Part model, mm, in its own coordinate system. A direction names the side the tool comes from. Coordinates: 2 decimals unless noted, no trailing zeros. Loops run counter-clockwise (first coordinate to the right, second up) from the corner with the lowest first, then second, coordinate; pieces in that order, holes last. Notation, with made-up numbers: M 66.5,10.5 L 113.5,10.5 A27 ccw 113.5,27.5 Z; hole C 26.25,69.5 d2. An arc over 180 degrees is marked long. Use a Markdown table: item, result. Add a question column.
1) Pull direction Y, two halves, no side cores. Call faces 1 (the flat face through (10, 4.758, 2)), 2 (the cylindrical face through (1.6, -28.8, 2)), 3 (the flat face through (3.167, -27.731, 2.366)): released by +Y, released by -Y, zero draft, split by the parting line, or undercut.
2) Band-saw the part on D-D (x = 9.5). List the corners of the cut face in (y, z), plus the area to 3 significant figures.
3) Pin check, flat tips, straight feed: pin 1 Ø10 at (x, y) = (16, -21.5) entering from +Z; pin 2 Ø2.5 at (y, z) = (-14.5, 2) entering from +X; pin 3 Ø2.5 at (y, z) = (-15, 3.5) entering from -X; pin 4 Ø4 at (x, y) = (1.5, 1) entering from -Z. Stop position of each tip, or through.
4) Band-saw the part on A-A (x = 0). List the corners of the cut face in (y, z).
5) Band-saw the part on B-B (z = 3.1). List the corners of the cut face in (x, y).
6) Tool access for faces 4 (the flat face through (0.754, -18, 2)), 5 (the flat face through (7.88, -15, 2)), 6 (the flat face through (2.554, -27, 2)), 7 (the flat face through (7.15, -11.65, 2.37)): list every direction of +Z, -Z, +X, -X, +Y, -Y with a clear straight run to the whole face (end or side of a thin tool).
7) Wall check: probe 1 along Y at (x, z) = (14.25, 2.75); probe 2 along X at (y, z) = (-17, 4.2); probe 3 along Y at (x, z) = (1.75, 0.9). Give the ranges that are in metal, low to high. Write a range as from..to.
8) Band-saw the part on C-C (y = -16). List the corners of the cut face in (x, z).
from build123d import *

# Parameters (mm, degrees)
SKETCH_1_R          = 5
SKETCH_1_R_2        = 2.5
EXTRUDE_1_DEPTH     = 4.8
SKETCH_3_R          = 1.825
CUT_EXTRUDE_1_DEPTH = 1.8
CUT_EXTRUDE_2_REACH = 36.158
SKETCH_4_R          = 0.1


with BuildPart() as part:
    # 스케치1 → 보스-돌출1 (new body)
    # profile 1 of 2: a face of its own
    with BuildSketch(Plane.XY):
        with BuildLine():
            ThreePointArc((5, 0), (0, -5), (-5, 0))
            Line((-5, 0), (-5, -2.326474397))
            Line((-5, -2.326474397), (0.754164722, -7.377840375))
            Line((0.754164722, -7.377840375), (0.754164722, -29.519890116))
            Line((0.754164722, -29.519890116), (2.889052882, -29.519890116))
            Line((2.889052882, -29.519890116), (3.452626944, -25.890848407))
            Line((3.452626944, -25.890848407), (7.880357437, -17.740939791))
            Line((7.880357437, -17.740939791), (7.880357437, -12.211059606))
            Line((7.880357437, -12.211059606), (6.40208237, -11.079255258))
            Line((6.40208237, -11.079255258), (6.40208237, -3.237610212))
            ThreePointArc((6.40208237, -3.237610212), (6.694975589, -2.530503431), (7.40208237, -2.237610212))
            Line((7.40208237, -2.237610212), (18.063612226, -2.237610212))
            Line((18.063612226, -2.237610212), (19.056002599, 4.757997197))
            Line((19.056002599, 4.757997197), (1.536705134, 4.757997197))
            ThreePointArc((1.536705134, 4.757997197), (4.04249463, 2.942488261), (5, 0))
        make_face()
    # profile 2 of 2: a face of its own
    with BuildSketch(Plane.XY):
        Circle(SKETCH_1_R)
        Circle(SKETCH_1_R_2, mode=Mode.SUBTRACT)
    extrude(amount=EXTRUDE_1_DEPTH)

    # 스케치3 → 컷-돌출1 (cut)
    with BuildSketch(Plane.ZY.offset(-0.754164722)):
        with Locations((2.4, -27.019890116)):
            Circle(SKETCH_3_R)
    extrude(amount=-CUT_EXTRUDE_1_DEPTH, mode=Mode.SUBTRACT)

    # 컷-돌출2: up to this plane
    cut_extrude_2_end = Plane(origin=(7.297372122, -1.133249487, 4.8), z_dir=(-0.9881554576984991, 0.15345615471746255, 0))
    # 스케치4 → 컷-돌출2 (cut, up to the surface)
    with BuildSketch(Plane.ZY.offset(-2.554164722), mode=Mode.PRIVATE) as cut_extrude_2_sk1:
        with Locations((2.4, -28.344890116)):
            Circle(SKETCH_4_R)
    cut_extrude_2_tool1 = split(extrude(cut_extrude_2_sk1.sketch, amount=-CUT_EXTRUDE_2_REACH, mode=Mode.PRIVATE), bisect_by=cut_extrude_2_end, keep=Keep.BOTH, mode=Mode.PRIVATE)
    add(cut_extrude_2_tool1.solids().sort_by_distance((2.554165, -28.34489, 2.4))[0], mode=Mode.SUBTRACT)


solid = part.part
Entries:
| question | item | result |
|---|---|---|
| 1 | face 1 | released by +Y |
| 1 | face 2 | undercut |
| 1 | face 3 | released by -Y |
| 2 | outline | M -2.24,0 L 4.76,0 L 4.76,4.8 L -2.24,4.8 Z |
| 2 | area | 33.6 mm2 |
| 3 | pin 1 | through |
| 3 | pin 2 | x = 7.88 |
| 3 | pin 3 | x = 0.75 |
| 3 | pin 4 | z = 0 |
| 4 | outline | M -6.72,0 L -2.5,0 L -2.5,4.8 L -6.72,4.8 Z; M 2.5,0 L 5,0 L 5,4.8 L 2.5,4.8 Z |
| 5 | outline | M -5,-2.33 L 0.75,-7.38 L 0.75,-25.33 L 2.55,-25.33 L 2.55,-28.71 L 0.75,-28.71 L 0.75,-29.52 L 2.89,-29.52 L 3.45,-25.89 L 7.88,-17.74 L 7.88,-12.21 L 6.4,-11.08 L 6.4,-3.24 A1 cw 7.4,-2.24 L 18.06,-2.24 L 19.06,4.76 L 1.54,4.76 A5 ccw -5,0 Z; hole C 0,0 d5 |
| 6 | face 4 | +Z, -Z, -X, -Y |
| 6 | face 5 | +Z, -Z, +X, -Y |
| 6 | face 6 | -X |
| 6 | face 7 | +Z, -Z, +X |
| 7 | probe 1 | -2.24..4.76 |
| 7 | probe 2 | 0.75..7.88 |
| 7 | probe 3 | -29.52..-28.06, -25.98..-1.79, 1.79..4.76 |
| 8 | outline | M 0.75,0 L 7.88,0 L 7.88,4.8 L 0.75,4.8 Z |
